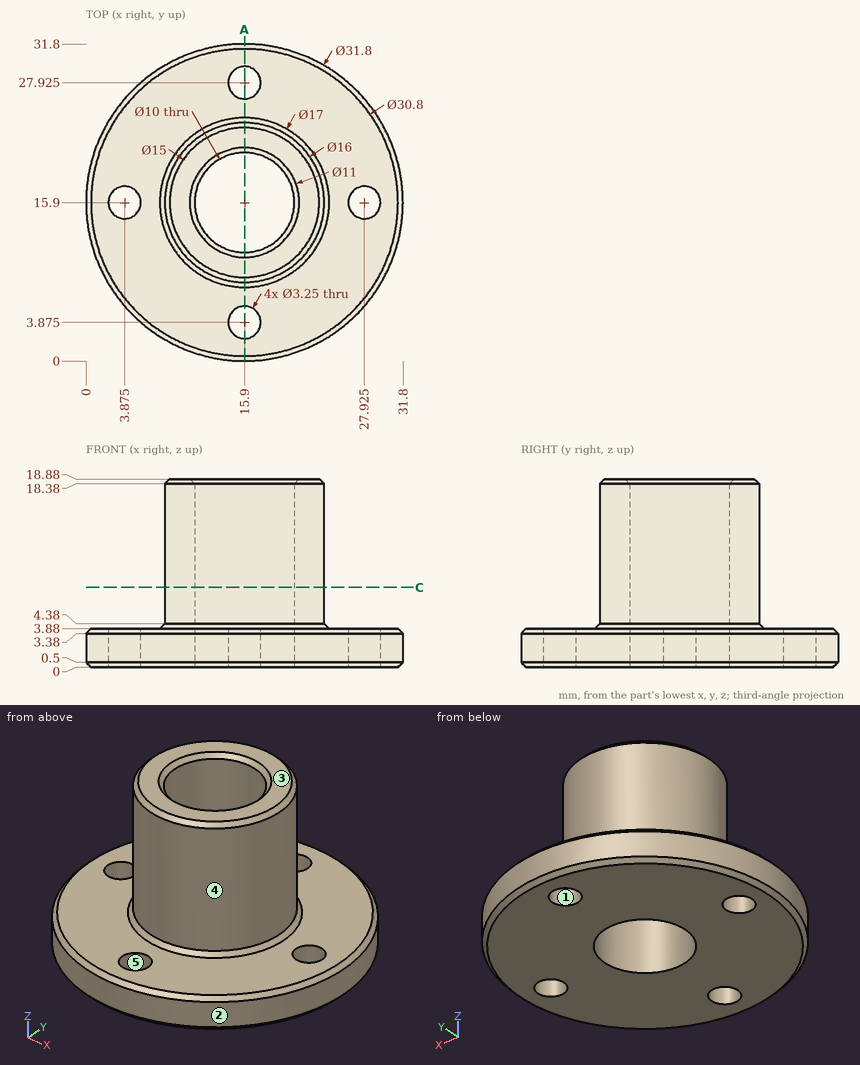
Could you check a few things on this drawing? It's one solid part, dimensions in mm from its lowest x, y, z. A direction names the side the tool comes from. Round coordinates to 2 decimals unless told otherwise and drop trailing zeros. Order: outer loops, then holes, each group sorted by start corner. A loop starts at its lowest first (then second) coordinate and runs counter-clockwise, first axis right, second up.
(1) Imagine slicing it at A-A (x = 15.9). Count the separate pieces of the cut face and the enclosed holes in it, plus the area to 3 significant figures.
Response values:
separate pieces: 4
enclosed holes: 0
area: 149 mm2
(2) Please list where these lines run through material, in increasing order: line 1 along Y through (x, z) = (15.9, 1); line 2 along Z through (x, y) = (22, 29.5); line 3 along X through (y, z) = (18, 15.75).
Response values:
line 1: y = 0 to 2.25, 5.5 to 10.9, 20.9 to 26.3, 29.55 to 31.8
line 2: z = 0 to 3.88
line 3: x = 8.18 to 11.36, 20.44 to 23.62
(3) I'm going to push flat-ended pins straight in: pin 1 (8 mm diameter, centred on x = 15.9, y = 15.9, fed in from -Z); pin 2 (3 mm diameter, centred on y = 7.5, z = 6.5, fed in from -X); pin 3 (4 mm diameter, centred on x = 15.9, y = 3.875, fed in from +Z); pin 4 (3 mm diameter, centred on y = 16, z = 12, fed in from -X). Where does each tip first touch, or does it pass through?
Response values:
pin 1: passes through
pin 2: stops at x = 11.85
pin 3: stops at z = 3.88
pin 4: stops at x = 7.9
(4) Imagine slicing it at C-C (z = 8). Write out the boundary of the cut face in (x, y), plus the area to 3 significant figures.
Response values:
outline: circle Ø16 at (15.9, 15.9); hole circle Ø10 at (15.9, 15.9)
area: 123 mm2
(5) If we mould it in two halves opening along Y, with no side actions, what happens to the marked faces 1, 2 and 3? For each: released by +Y, released by -Y, zero draft, split by the parting line, or undercut.
Response values:
face 1: undercut
face 2: split by the parting line
face 3: zero draft
(6) Which directions (+Z, -Z, +X, -X, +Y, -Y) give clear straight access to the entire face, cutting with the end or side of a thin tool? Please do the marked faces 4 and 5.
Response values:
face 4: +Z
face 5: +Z, -Z
